```python
from build123d import *

# Parameters (mm, degrees)
BOSS_EXTRUDE1_DEPTH = 2
BOSS_EXTRUDE2_DEPTH = 6
SKETCH24_R          = 3.9
BOSS_EXTRUDE5_DEPTH = 2.3
SKETCH30_W          = 2.408612022
SKETCH30_H          = 1.324178481
CUT_EXTRUDE12_DEPTH = 8
CUT_EXTRUDE11_DEPTH = 5.3
FILLET1_R           = 1.5
SKETCH34_R          = 0.75
CUT_EXTRUDE13_DEPTH = 8
SKETCH35_R          = 0.75
CUT_EXTRUDE14_DEPTH = 4
SKETCH36_R          = 0.95
CUT_EXTRUDE15_DEPTH = 8
SKETCH37_R          = 2
CUT_EXTRUDE16_DEPTH = 2.5
SKETCH38_W          = 3
SKETCH38_H          = 1.25
CUT_EXTRUDE17_DEPTH = 3.6


with BuildPart() as part:
    # Sketch2 → Boss-Extrude1 (new body)
    with BuildSketch(Plane.XY):
        with BuildLine():
            Line((-2.5, 7.5), (-16.7, 7.5))
            Line((-16.7, 7.5), (-20.7, 3.793442666))
            Line((-20.7, 3.793442666), (-20.7, -4.031648778))
            Line((-20.7, -4.031648778), (-15.7, -7.5))
            Line((-15.7, -7.5), (-6.7, -7.5))
            Line((-6.7, -7.5), (-4.2, -5.6))
            ThreePointArc((-4.2, -5.6), (3.130495168, -6.260990337), (7, 0))
            ThreePointArc((7, 0), (4.949747468, 4.949747468), (0, 7))
            Line((0, 7), (0, 7.5))
            Line((0, 7.5), (-2.5, 7.5))
        make_face()
    extrude(amount=BOSS_EXTRUDE1_DEPTH)

    # Sketch4 → Boss-Extrude2 (add)
    with BuildSketch(Plane.XY.offset(2)):
        Polygon((-15.7, -7.5), (-6.7, -7.5), (-6.759079174, -4.5), (-7.7, -4.5), (-7.7, 2), (-5.5, 2), (-5.5, 5.3), (-2.5, 5.3), (-2.5, 7.5), (-16.7, 7.5), (-20.7, 3.793442666), (-20.7, -4.031648778), align=None)
    extrude(amount=BOSS_EXTRUDE2_DEPTH)

    # Sketch24 → Boss-Extrude5 (add)
    with BuildSketch(Plane.XY.offset(2)):
        Circle(SKETCH24_R)
    extrude(amount=BOSS_EXTRUDE5_DEPTH)

    # Sketch30 → Cut-Extrude12 (cut)
    with BuildSketch(Plane(origin=(-5.5, 0, 0), x_dir=(0, 0, -1), z_dir=(1, 0, 0))):
        with Locations((-3.261593395, 4.63791076)):
            Rectangle(SKETCH30_W, SKETCH30_H)
    extrude(amount=-CUT_EXTRUDE12_DEPTH, mode=Mode.SUBTRACT)

    # Sketch28 → Cut-Extrude11 (cut, through all)
    with BuildSketch(Plane.XY.offset(4.3)):
        with BuildLine():
            Line((-1, 1.732050808), (-1, -1.732050808))
            ThreePointArc((-1, -1.732050808), (2, 0), (-1, 1.732050808))
        make_face()
    extrude(amount=-CUT_EXTRUDE11_DEPTH, mode=Mode.SUBTRACT)

    # Fillet1
    fillet1_edges = [part.edges().sort_by_distance(p)[0] for p in [
        (-11.2, -7.5, 0),
        (-8.35, 7.5, 0),
        (-18.7, 5.646721333, 0),
        (-18.2, -5.765824389, 0),
        (-20.7, -0.119103056, 0),
        (-15.7, -7.5, 4),
        (-20.7, -4.031648778, 4),
        (-20.7, 3.793442666, 4),
        (-16.7, 7.5, 4),
    ]]
    fillet(fillet1_edges, radius=FILLET1_R)

    # Sketch34 → Cut-Extrude13 (cut, along a direction that is not the sketch's normal)
    with BuildSketch(Plane.XZ.offset(-2)):
        with Locations((-7, 8)):
            Circle(SKETCH34_R)
    extrude(amount=-CUT_EXTRUDE13_DEPTH, dir=(0.668583388, -0.743637179, 0), mode=Mode.SUBTRACT)

    # Sketch35 → Cut-Extrude14 (cut, symmetric, along a direction that is not the sketch's normal)
    with BuildSketch(Plane(origin=(0, -4.5, 0), x_dir=(1, 0, 0), z_dir=(0, 1, 0))):
        with Locations((-8.259079174, -8)):
            Circle(SKETCH35_R)
    extrude(amount=CUT_EXTRUDE14_DEPTH, dir=(0.599919418, 0.80006043, 0), both=True, mode=Mode.SUBTRACT)

    # Sketch36 → Cut-Extrude15 (cut)
    with BuildSketch(Plane.XY.offset(8)):
        with Locations((-11.7, 0)):
            Circle(SKETCH36_R)
        with Locations((-16.7, 0)):
            Circle(SKETCH36_R)
    extrude(amount=-CUT_EXTRUDE15_DEPTH, mode=Mode.SUBTRACT)

    # Sketch37 → Cut-Extrude16 (cut)
    with BuildSketch(Plane(origin=(0, 0, 0), x_dir=(-1, 0, 0), z_dir=(0, 0, -1))):
        with Locations((11.7, 0)):
            Circle(SKETCH37_R)
        with Locations((16.7, 0)):
            Circle(SKETCH37_R)
    extrude(amount=-CUT_EXTRUDE16_DEPTH, mode=Mode.SUBTRACT)

    # Sketch38 → Cut-Extrude17 (cut)
    with BuildSketch(Plane.XY.offset(8)):
        with Locations((-4, 5.925)):
            Rectangle(SKETCH38_W, SKETCH38_H)
    extrude(amount=-CUT_EXTRUDE17_DEPTH, mode=Mode.SUBTRACT)


with BuildPart() as body_2:
    # Split2: the piece on the far side of the plane
    add(part.part)
    split(bisect_by=Plane.XY.offset(4.4), keep=Keep.BOTTOM)


with BuildPart() as part_1:
    add(part.part)

    # Split2
    split(bisect_by=Plane.XY.offset(4.4), keep=Keep.TOP)


with BuildPart() as body_3:
    # Mirror2: mirrored copy
    add(body_2.part.mirror(Plane.XY.offset(8)))


solid = body_3.part
```
Design review of the part built by this model. Coordinates are the model's own, in mm. A direction names the side the tool comes from. Round coordinates to 2 decimals unless told otherwise and drop trailing zeros. Write each loop counter-clockwise with the first axis right and the second up, starting at its lowest first coordinate (ties: lowest second). Pieces come first, ordered by that corner, then holes. Notation, with made-up numbers: (88, 80) -> (101, 80) arc R12 ccw to (101, 100) -> close; hole circle Ø7 at (-33.75, 63.5). An arc over 180 degrees is marked (long way). Write item = value, one per line. Start each with the question number.
1) Take a section at D-D, the plane y = 1.25. State the section outline as (x, z) points.
2) Take a section at A-A, the plane x = -11.7. State the section outline as (y, z) points.
3) Mouldability with a two-part tool opening along X and no side actions: class faces 1 (the face through (-18, 0, 13.5)), 2 (the face through (-20.524, -3.951, 13.07)), 3 (the face through (-9, 3.976, 13)) as +X half, -X half, draft (parallel to the pull), parting line (faces both ways), or undercut.
4) Take a section at B-B, the plane y = -0.5. Count the separate pieces of the cut face and the enclosed holes in it, plus the area to 3 significant figures.
5) Take a section at C-C, the plane z = 14.9. State the section outline as (x, y) points.
6) Wall thickness on probe 1 along Y at (x, z) = (-7, 12); probe 2 along X at (y, z) = (-0.25, 15.55); probe 3 along X at (y, z) = (0.25, 14.65): over which ranges is each line inside the solid? List them lowest first. Write a range as from..to.
7) Tool access review of faces 4 (the face through (-12.623, -1.774, 14.768)), 5 (the face through (-13.5, 5, 13)), 6 (the face through (-2.87, 2.64, 12.87)): name each direction out of +Z, -Z, +X, -X, +Y, -Y from which nothing blocks a thin tool from reaching the whole face with its end or side.
8) Clearance check with flat-ended pins moving along their axes: pin 1 (8.5 mm diameter, centred on x = -1.5, y = -1, fed in from -Z); pin 2 (2.5 mm diameter, centred on y = 7, z = 12.5, fed in from +X); pin 3 (2 mm diameter, centred on x = -11.7, y = 0, fed in from +Z). State where each tip first meets the part, or that it passes through.
Results list:
q1.outline = (-20.7, 11.6) -> (-7.7, 11.6) -> (-7.7, 14) -> (-3.69, 14) -> (-3.69, 11.7) -> (-1, 11.7) -> (-1, 16) -> (-10.14, 16) -> (-10.14, 13.5) -> (-13.26, 13.5) -> (-13.26, 16) -> (-15.14, 16) -> (-15.14, 13.5) -> (-18.26, 13.5) -> (-18.26, 16) -> (-19.2, 16) arc R1.5 ccw to (-20.7, 14.5) -> close; (1.56, 11.7) -> (3.69, 11.7) -> (3.69, 14) -> (6.89, 14) -> (6.89, 16) -> (1.56, 16) -> close
q2.outline = (-7.5, 11.6) -> (-0.95, 11.6) -> (-0.95, 13.5) -> (-2, 13.5) -> (-2, 16) -> (-6, 16) arc R1.5 ccw to (-7.5, 14.5) -> close; (0.95, 11.6) -> (3.98, 11.6) -> (3.98, 13.94) -> (5.3, 13.94) -> (5.3, 11.6) -> (7.5, 11.6) -> (7.5, 14.5) arc R1.5 ccw to (6, 16) -> (2, 16) -> (2, 13.5) -> (0.95, 13.5) -> close
q3.face_1 = undercut
q3.face_2 = -X half
q3.face_3 = draft
q4.separate_pieces = 4
q4.enclosed_holes = 0
q4.area = 65.7 mm²
q5.outline = (-20.65, -3.25) arc R1.45 ccw to (-20.02, -4.43) -> (-16.05, -7.19) arc R1.45 ccw to (-15.23, -7.45) -> (-6.63, -7.45) -> (-4.2, -5.6) arc R7 ccw (long way) to (0, 7) -> (0, 7.45) -> (-16.11, 7.45) arc R1.45 ccw to (-17.09, 7.06) -> (-20.18, 4.2) arc R1.45 ccw to (-20.65, 3.14) -> close; hole circle Ø4 at (-16.7, 0); hole circle Ø4 at (-11.7, 0); hole (-1, -1.73) arc R2 ccw (long way) to (-1, 1.73) -> close
q6.probe_1 = -7.5..-4.5, 2..3.98, 5.3..7.5
q6.probe_2 = -20.27..-18.68, -14.72..-13.68, -9.72..-1, 1.98..7
q6.probe_3 = -20.69..-18.68, -14.72..-13.68, -9.72..-1, 1.98..7
q7.face_4 = +Z
q7.face_5 = -Z, +X
q7.face_6 = -Z
q8.pin_1 = 11.7
q8.pin_2 = -2.5
q8.pin_3 = 13.5
